Drawing for the job (mm, zero at the part's lowest x, y, z). A direction names the side the tool comes from. Coordinates: 2 decimals unless noted, no trailing zeros. Loops run counter-clockwise (first coordinate to the right, second up) from the corner with the lowest first, then second, coordinate; pieces in that order, holes last. Notation, with made-up numbers: (80.25, 83) - (110.25, 83) arc R8 cw to (110.25, 88) - close; hole circle Ø6 at (4, 19). An arc over 180 degrees is marked (long way). Put each result on its own line as item: value.
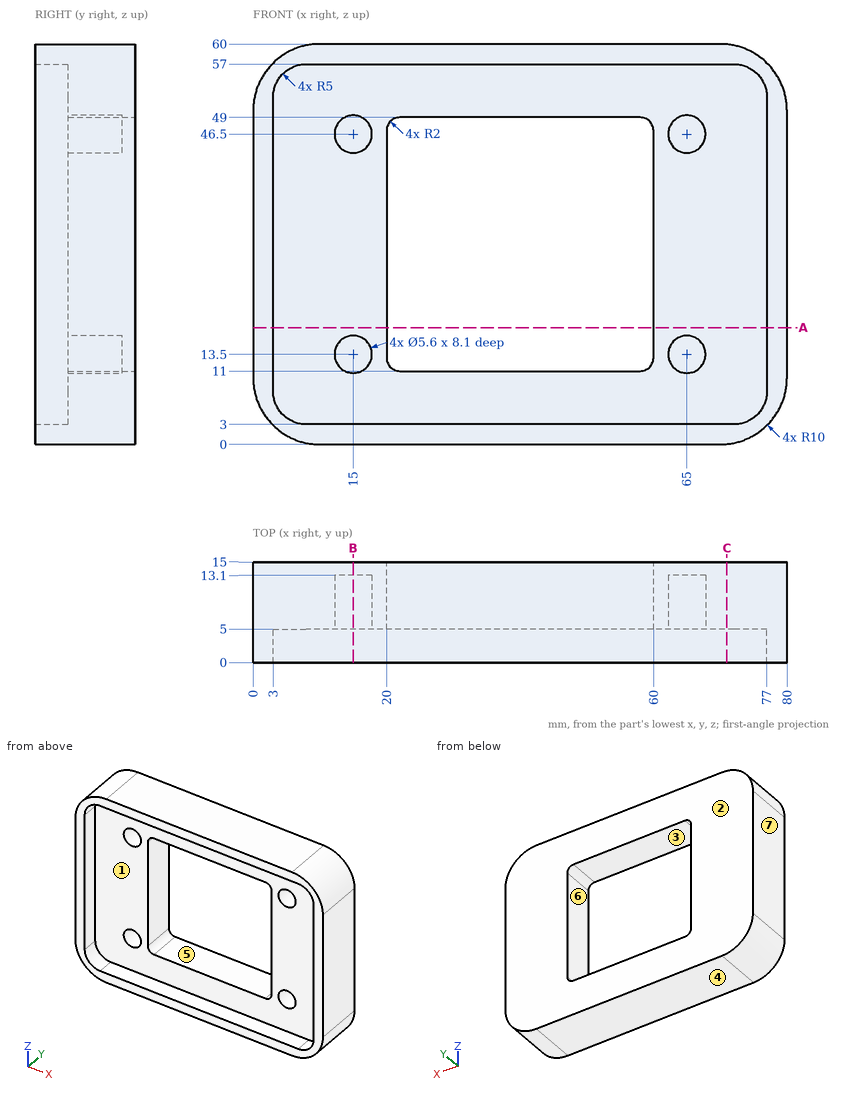
Q1. Slice it at B-B, the plane x = 15. Give the cut face in (y, z), then the cut area to 3 significant figures.
Determined:
outline: (0, 0) - (15, 0) - (15, 60) - (0, 60) - (0, 57) - (5, 57) - (5, 49.3) - (13.1, 49.3) - (13.1, 43.7) - (5, 43.7) - (5, 16.3) - (13.1, 16.3) - (13.1, 10.7) - (5, 10.7) - (5, 3) - (0, 3) - close
area: 539 mm2
Q2. Mould opens along Z. For the marked faces 4, 5, 6 and 7 say: +Z half, -Z half, draft (parallel to the pull), parting line (faces both ways), or undercut.
Determined:
face 4: -Z half
face 5: undercut
face 6: undercut
face 7: draft
Q3. Pin check, flat tips, straight feed: pin 1 Ø4.5 at (x, z) = (65, 46) entering from -Y; pin 2 Ø3 at (x, z) = (14, 45) entering from -Y. Stop position of each tip, or through.
Determined:
pin 1: y = 13.1
pin 2: y = 5
Q4. Slice it at A-A, the plane z = 17.5. Give the cut face in (x, y), then the cut area to 3 significant figures.
Determined:
outline: (0, 0) - (3, 0) - (3, 5) - (20, 5) - (20, 15) - (0, 15) - close; (60, 5) - (77, 5) - (77, 0) - (80, 0) - (80, 15) - (60, 15) - close
area: 430 mm2
Q5. Tool access for the marked faces 1, 2 and 3: list every direction of +Z, -Z, +X, -X, +Y, -Y with a clear straight run to the whole face (end or side of a thin tool).
Determined:
face 1: -Y
face 2: +Z, -Z, +X, -X, +Y
face 3: +Y, -Y
Q6. Slice it at C-C, the plane x = 71. Give the cut face in (y, z).
Determined:
outline: (0, 0.05) - (15, 0.05) - (15, 59.95) - (0, 59.95) - (0, 57) - (5, 57) - (5, 3) - (0, 3) - close
Q7. Wall check: L1, parallel to X at y = 9.25, z = 13.5; L2, parallel to Z at x = 50, y = 8.5; L3, parallel to X at y = 13.5, z = 27. Give the ranges that are in metal, low to high. Write a range as from..to.
Determined:
L1: 0..12.2, 17.8..20, 60..62.2, 67.8..80
L2: 0..11, 49..60
L3: 0..20, 60..80
